CAD build for the part. Positions are in the model's coordinates, mm. Face numbers are marked on the shaded views. A direction names the side the tool comes from. Round coordinates to 2 decimals unless told otherwise and drop trailing zeros. Write each loop counter-clockwise with the first axis right and the second up, starting at its lowest first coordinate (ties: lowest second). Pieces come first, ordered by that corner, then holes. Notation, with made-up numbers: (56.5, -26.5) - (90.5, -26.5) arc R8 cw to (90.5, -22.5) - close; hole circle Ø4 at (-16.75, 10). An arc over 180 degrees is marked (long way). Put each result on its own line as item: value. Start each with the question number.
Item 1: Mould opens along X. For the marked faces 1, 2, 3 and 4 say: released by +X, released by -X, zero draft, split by the parting line, or undercut.
Item 2: Pin check, flat tips, straight feed: pin 1 Ø7.5 at (x, y) = (122.5, -212) entering from -Z; pin 2 Ø7.5 at (x, z) = (220.5, 165) entering from +Y; pin 3 Ø10 at (x, z) = (99.5, 320) entering from -Y; pin 4 Ø4.5 at (x, z) = (230.5, -5.5) entering from -Y. Stop position of each tip, or through.
Item 3: Cut at B-B (y = -56). Give the cut face in (x, z).
Item 4: Cut at C-C (z = 58.5). Give the cut face in (x, y).
Item 5: 3-axis set-ups, long thin cutter, end or side, ignore diameter. For the marked faces 5 and 6: which of +Z, -Z, +X, -X, +Y, -Y reach the whole face in a straight line?
Item 6: Drill centre lines: line 1 (Z direction, x = 18, y = -201); line 2 (X direction, y = -42, z = 218.5); line 3 (Y direction, x = 36, z = 244.5). Where is each one in solid material? Low to high. Write a range as from..to.
Item 7: Cut at A-A (x = 279). Give the cut face in (y, z), and give its area (4 significant figures).
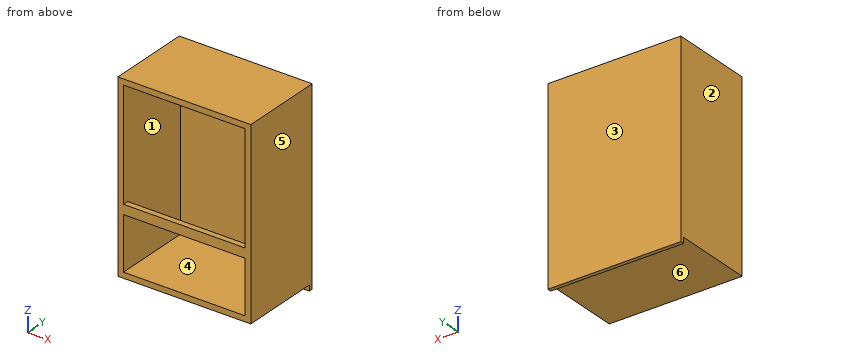
```python
from build123d import *

# Parameters (mm, degrees)
F0_W     = 350
F0_H     = 485
F1_DEPTH = 220
F2_T     = -15
F3_W     = 320
F3_H     = 25
F4_DEPTH = 15
F5_W     = 350
F5_H     = 10
F6_DEPTH = 15


with BuildPart() as f1:
    # F0 (on Front) → F1 (new body)
    with BuildSketch(Plane.XZ):
        with Locations((175, 242.5)):
            Rectangle(F0_W, F0_H)
    extrude(amount=F1_DEPTH)

    # F2
    f2_openings = [f1.faces().sort_by_distance(p)[0] for p in [
        (175, -220, 242.5),
    ]]
    offset(amount=F2_T, openings=f2_openings)

    # F3 (on face) → F4 (join)
    with BuildSketch(Plane.XZ.offset(220)):
        with Locations((175, 167.5)):
            Rectangle(F3_W, F3_H)
    extrude(amount=-F4_DEPTH)

    # F5 (on face) → F6 (join)
    with BuildSketch(Plane(origin=(0, 0, 0), x_dir=(1, 0, 0), z_dir=(0, 0, -1))):
        with Locations((175, 5)):
            Rectangle(F5_W, F5_H)
    extrude(amount=F6_DEPTH)


solid = f1.part
```
Output values:
1. face 1: undercut
1. face 2: released by -X
1. face 3: zero draft
1. face 4: undercut
2. pin 1: z = 0
2. pin 2: y = 0
2. pin 3: y = -15
2. pin 4: y = -10
3. outline: (0, 0) - (350, 0) - (350, 485) - (0, 485) - close; hole (15, 15) - (335, 15) - (335, 470) - (15, 470) - close
4. outline: (0, -220) - (15, -220) - (15, -15) - (335, -15) - (335, -220) - (350, -220) - (350, 0) - (0, 0) - close
5. face 5: +Z, -Z, +X, +Y, -Y
5. face 6: -Z, +X, -X, -Y
6. line 1: 0..15, 470..485
6. line 2: 0..15, 335..350
6. line 3: -15..0
7. outline: (-220, 0) - (-10, 0) - (-10, -15) - (0, -15) - (0, 485) - (-220, 485) - (-220, 470) - (-15, 470) - (-15, 15) - (-220, 15) - close; (-220, 155) - (-205, 155) - (-205, 180) - (-220, 180) - close
7. area: 13,950 mm2
